from build123d import *

# Parameters (mm, degrees)
SKETCH1_R           = 2.5
SKETCH1_R_2         = 11
SKETCH1_R_3         = 1.75
BOSS_EXTRUDE1_DEPTH = 6


with BuildPart() as part:
    # Sketch1 → Boss-Extrude1 (new body)
    with BuildSketch(Plane(origin=(0, 0, 0), x_dir=(0, 0, -1), z_dir=(1, 0, 0))):
        Polygon((0, 0), (400, 0), (400, 400), (200, 400), (0, 60), align=None)
        with Locations((30, 42)):
            Circle(SKETCH1_R, mode=Mode.SUBTRACT)
        with Locations(Location((30, 18, 0), (0, 0, 180))):
            Circle(SKETCH1_R, mode=Mode.SUBTRACT)
        with Locations((370, 18)):
            Circle(SKETCH1_R, mode=Mode.SUBTRACT)
        with Locations(Location((370, 42, 0), (0, 0, 180))):
            Circle(SKETCH1_R, mode=Mode.SUBTRACT)
        with Locations((310, 350)):
            Circle(SKETCH1_R, mode=Mode.SUBTRACT)
        with Locations((310, 250)):
            Circle(SKETCH1_R, mode=Mode.SUBTRACT)
        with Locations((320, 300)):
            Circle(SKETCH1_R_2, mode=Mode.SUBTRACT)
        with Locations((335.5, 315.5)):
            Circle(SKETCH1_R_3, mode=Mode.SUBTRACT)
        with Locations(Location((304.5, 315.5, 0), (0, 0, 180))):
            Circle(SKETCH1_R_3, mode=Mode.SUBTRACT)
        with Locations((304.5, 284.5)):
            Circle(SKETCH1_R_3, mode=Mode.SUBTRACT)
        with Locations(Location((335.5, 284.5, 0), (0, 0, 180))):
            Circle(SKETCH1_R_3, mode=Mode.SUBTRACT)
    extrude(amount=BOSS_EXTRUDE1_DEPTH)


solid = part.part
Verification items for the finished model (mm, model axes). Round coordinates to 2 decimals unless told otherwise and drop trailing zeros. Write each loop counter-clockwise with the first axis right and the second up, starting at its lowest first coordinate (ties: lowest second). Pieces come first, ordered by that corner, then holes.
(1) Section check C-C (y = 89.5). Enter the section's corners in (x, z), plus the area to 3 significant figures.
Returned:
outline: (0, -400) - (6, -400) - (6, -17.35) - (0, -17.35) - close
area: 2,300 mm2
(2) Depth check by flat-ended pin: pin 1 Ø6 at (y, z) = (338, -352.5) entering from -X; pin 2 Ø3 at (x, z) = (4, -175.5) entering from +Y; pin 3 Ø2 at (x, y) = (1, 313.5) entering from +Z. Enter the tip coordinate at first touch or a pass-through.
Returned:
pin 1: stops at x = 0
pin 2: stops at y = 360.9
pin 3: stops at z = -148.53
(3) Section check A-A (x = 4.9). Give the number of separate pieces and of enclosed holes in the cut face, plus the area to 3 significant figures.
Returned:
separate pieces: 1
enclosed holes: 11
area: 125,000 mm2
(4) Section check B-B (z = -83). Enter the section's corners in (x, y).
Returned:
outline: (0, 0) - (6, 0) - (6, 201.1) - (0, 201.1) - close
(5) Mould release check, pull along Z, two halves, no side actions. Record for faces 1 (the flat face through (2.96, 232.38, -101.4)), 2 (the cylindrical face through (3, 300, -309)), 3 (the flat face through (6, 158, -242)): pulls with the +Z half, pulls with the -Z half, needs draft (parallel to the pull), parting line crosses it, or undercut.
Returned:
face 1: pulls with the +Z half
face 2: undercut
face 3: needs draft
(6) Material ranges on line 1 (Y direction, x = 1.65, z = -370); line 2 (Y direction, x = 2.2, z = -304.5); line 3 (Y direction, x = 4.65, z = -319), recorded low to high.
Returned:
line 1: y = 0 to 15.5, 20.5 to 39.5, 44.5 to 400
line 2: y = 0 to 282.75, 286.25 to 313.75, 317.25 to 400
line 3: y = 0 to 289.05, 310.95 to 400
